Check sheet for the modelled part. Datum: model origin and axes. Units: mm. Round coordinates to 2 decimals unless told otherwise and drop trailing zeros. Order: outer loops, then holes, each group sorted by start corner. A loop starts at its lowest first (then second) coordinate and runs counter-clockwise, first axis right, second up.
from build123d import *

# Parameters (mm, degrees)
F0_W     = 60
F0_H     = 20
F1_DEPTH = 900
F3_R     = 3
F4_DEPTH = 12
F5_R     = 3
F6_DEPTH = 12
F7_W     = 6
F7_H     = 3
F8_DEPTH = 900


with BuildPart() as f1:
    # F0 (on Top) → F1 (new body)
    with BuildSketch(Plane.XY):
        with Locations((30, 10)):
            Rectangle(F0_W, F0_H)
    extrude(amount=F1_DEPTH)

    # F3 (on face) → F4 (cut)
    with BuildSketch(Plane(origin=(0, 0, 0), x_dir=(1, 0, 0), z_dir=(0, 0, -1))):
        with Locations((30, -10)):
            Circle(F3_R)
    extrude(amount=-F4_DEPTH, mode=Mode.SUBTRACT)

    # F5 (on face) → F6 (cut)
    with BuildSketch(Plane.XY.offset(900)):
        with Locations((30, 10)):
            Circle(F5_R)
    extrude(amount=-F6_DEPTH, mode=Mode.SUBTRACT)

    # F7 (on face) → F8 (cut)
    with BuildSketch(Plane.XY.offset(900)):
        with Locations((3, 1.5)):
            Rectangle(F7_W, F7_H)
    extrude(amount=-F8_DEPTH, mode=Mode.SUBTRACT)


solid = f1.part
1) Gauge pin test, flat ends, axial feed: pin 1 (3.5 mm diameter, centred on y = 1, z = 556.5, fed in from -X); pin 2 (1.8 mm diameter, centred on x = 3.5, z = 560.5, fed in from -Y); pin 3 (3.5 mm diameter, centred on x = 30, y = 10, fed in from +Z). Record the tip position at first contact, or that the pin passes through.
2) Sectioned sample at A-A on z = 655. Record the cut outline in (x, y).
3) Scan lines: line 1 (Y direction, x = 30, z = 6); line 2 (X direction, y = 10, z = 3.5); line 3 (X direction, y = 1.5, z = 742.5). Record each from-to range of solid material in increasing order.
Values found:
1. pin 1: stops at x = 6
1. pin 2: stops at y = 3
1. pin 3: stops at z = 888
2. outline: (0, 3) - (6, 3) - (6, 0) - (60, 0) - (60, 20) - (0, 20) - close
3. line 1: y = 0 to 7, 13 to 20
3. line 2: x = 0 to 27, 33 to 60
3. line 3: x = 6 to 60
